Check sheet for the modelled part. Datum: model origin and axes. Units: mm. Face numbers are marked on the shaded views. A direction names the side the tool comes from. Coordinates: 2 decimals unless noted, no trailing zeros. Write each loop counter-clockwise with the first axis right and the second up, starting at its lowest first coordinate (ties: lowest second). Pieces come first, ordered by that corner, then holes. Notation, with made-up numbers: (23, -10) - (82, -10) arc R19 ccw to (82, 12) - close; hole circle Ø10 at (-39.5, 82). An arc over 180 degrees is marked (long way). Use one line per item in the form item = value. Start each with the question number.
1. Go/stop test with flat-tipped pins: pin 1 Ø0.8 at (x, y) = (-25.5, -4.5) entering from +Z; pin 2 Ø1.1 at (x, y) = (-2, -4.5) entering from +Z; pin 3 Ø0.5 at (y, z) = (-4.5, 0.5) entering from +X; pin 4 Ø0.8 at (y, z) = (-4.5, 0.5) entering from -X. Record where each tip stops, or that it passes through.
2. Scan lines: line 1 along X through (y, z) = (2.9, 4); line 2 along Y through (x, z) = (29.5, 5); line 3 along Y through (x, z) = (37, 7.25). Record each from-to range of solid material in increasing order.
3. Tool access check on the marked faces 1, 2 and 3. Record the directions out of +Z, -Z, +X, -X, +Y, -Y that give a thin tool (end or side, any length) a straight path to the whole face; none if there is none.
4. Cross-section at B-B on x = 11. Record the boundary of the cut face in (y, z), then the cut area to 3 significant figures.
5. Cross-section at C-C on y = -1. Record the boundary of the cut face in (x, z).
6. Cross-section at A-A on z = 4. Record the boundary of the cut face in (x, y).
```python
from build123d import *

# Parameters (mm, degrees)
SKETCH1_W           = 72.5
SKETCH1_H           = 8
BOSS_EXTRUDE1_DEPTH = 8
SKETCH2_W           = 4
SKETCH2_H           = 1
EXTRUDE_THIN1_DEPTH = 1
LPATTERN1_COUNT     = 8
LPATTERN1_PITCH     = 4.5
LPATTERN1_COL_COUNT = 9
LPATTERN1_COL_PITCH = 4.5
SKETCH3_W           = 8
SKETCH3_H           = 2.3
BOSS_EXTRUDE2_DEPTH = 12
SKETCH4_OUTSIDE_W   = 117.95
SKETCH4_OUTSIDE_H   = 29.45
SKETCH4_OUTSIDE_R   = 2.5
CUT_EXTRUDE1_DEPTH  = 50.729895435
CHAMFER1_SIZE       = 0.5


with BuildPart() as part:
    # Sketch1 → Boss-Extrude1 (new body)
    with BuildSketch(Plane.XY):
        Rectangle(SKETCH1_W, SKETCH1_H)
    extrude(amount=BOSS_EXTRUDE1_DEPTH)

    # Sketch2 → Extrude-Thin1 (add)
    with BuildSketch(Plane.XZ.offset(4)):
        with Locations((-2.25, 0.5)):
            Rectangle(SKETCH2_W, SKETCH2_H)
    extrude_thin1 = extrude(amount=EXTRUDE_THIN1_DEPTH)

    # LPattern1: Extrude-Thin1 ×8
    with Locations(*[(-i * LPATTERN1_PITCH, 0, 0) for i in range(1, LPATTERN1_COUNT)]):
        add(extrude_thin1)

    # LPattern1 col: Extrude-Thin1 ×9
    with Locations(*[(i * LPATTERN1_COL_PITCH, 0, 0) for i in range(1, LPATTERN1_COL_COUNT)]):
        add(extrude_thin1)

    # Sketch3 → Boss-Extrude2 (add)
    with BuildSketch(Plane(origin=(36.25, 0, 0), x_dir=(0, 0, -1), z_dir=(1, 0, 0))):
        with Locations((-4, 2.85)):
            Rectangle(SKETCH3_W, SKETCH3_H)
    boss_extrude2 = extrude(amount=BOSS_EXTRUDE2_DEPTH)

    # Mirror1: Boss-Extrude2 across plane
    add(boss_extrude2.mirror(Plane(origin=(0, 0, 0), x_dir=(0, 0, 1), z_dir=(1, 0, 0))))

    # Sketch4 outside → Cut-Extrude1 (cut, through all)
    # profile 1 of 3: a face of its own
    with BuildSketch(Plane(origin=(0, 4, 0), x_dir=(1, 0, 0), z_dir=(0, 1, 0))):
        with Locations((0, -4)):
            Rectangle(SKETCH4_OUTSIDE_W, SKETCH4_OUTSIDE_H)
        with BuildLine():
            Line((-42.25, 0), (42.25, 0))
            ThreePointArc((42.25, 0), (46.25, -4), (42.25, -8))
            Line((42.25, -8), (-42.25, -8))
            ThreePointArc((-42.25, -8), (-46.25, -4), (-42.25, 0))
        make_face(mode=Mode.SUBTRACT)
    # profile 2 of 3: a face of its own
    with BuildSketch(Plane(origin=(0, 4, 0), x_dir=(1, 0, 0), z_dir=(0, 1, 0))):
        with Locations(Location((-42.25, -4, 0), (0, 0, 270))):
            Circle(SKETCH4_OUTSIDE_R)
    # profile 3 of 3: a face of its own
    with BuildSketch(Plane(origin=(0, 4, 0), x_dir=(1, 0, 0), z_dir=(0, 1, 0))):
        with Locations(Location((42.25, -4, 0), (0, 0, 270))):
            Circle(SKETCH4_OUTSIDE_R)
    extrude(amount=-CUT_EXTRUDE1_DEPTH, mode=Mode.SUBTRACT)

    # Chamfer1
    chamfer1_edges = [part.edges().sort_by_distance(p)[0] for p in [
        (42.25, 1.7, 1.5),
        (42.25, 4, 1.5),
        (-42.25, 1.7, 1.5),
        (-42.25, 4, 1.5),
    ]]
    chamfer(chamfer1_edges, length=CHAMFER1_SIZE)


solid = part.part
```
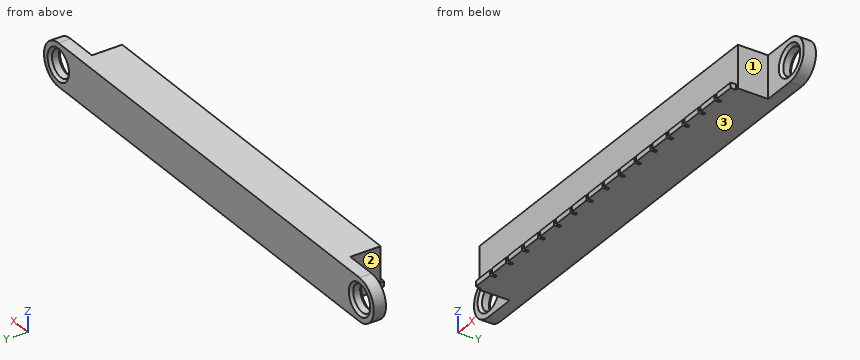
Final values:
q1.pin_1 = 1
q1.pin_2 = 8
q1.pin_3 = 35.75
q1.pin_4 = -35.75
q2.line_1 = -46.25 to -44.75, -39.75 to 39.75, 44.75 to 46.25
q2.line_2 = -4 to 4
q2.line_3 = 1.7 to 4
q3.face_1 = +Z, -Z, +X, -Y
q3.face_2 = +Z, -Z, -X, -Y
q3.face_3 = -Z, +X, -X, +Y, -Y
q4.outline = (-5, 0) - (4, 0) - (4, 8) - (-4, 8) - (-4, 1) - (-5, 1) - close
q4.area = 65.0 mm²
q5.outline = (-36.25, 0) - (36.25, 0) - (36.25, 8) - (-36.25, 8) - close
q6.outline = (-46.25, 1.7) - (-45.25, 1.7) - (-44.75, 2.2) - (-44.75, 3.5) - (-45.25, 4) - (-46.25, 4) - close; (-39.75, 2.2) - (-39.25, 1.7) - (-36.25, 1.7) - (-36.25, -4) - (36.25, -4) - (36.25, 1.7) - (39.25, 1.7) - (39.75, 2.2) - (39.75, 3.5) - (39.25, 4) - (-39.25, 4) - (-39.75, 3.5) - close; (44.75, 2.2) - (45.25, 1.7) - (46.25, 1.7) - (46.25, 4) - (45.25, 4) - (44.75, 3.5) - close
